Verification items for the finished model (mm, model axes). A direction names the side the tool comes from. Coordinates: 2 decimals unless noted, no trailing zeros. Order: outer loops, then holes, each group sorted by start corner. A loop starts at its lowest first (then second) coordinate and runs counter-clockwise, first axis right, second up. Notation, with made-up numbers: (-27.5, -12.75) -> (24.5, -12.75) arc R16 cw to (24.5, 13.25) -> close; hole circle Ø10 at (56, 72.25). An arc over 180 degrees is marked (long way). Use CSV: the item, a comma, the result in double quotes. Start each with the question number.
1) Tool access check on faces 1 (the flat face through (6, 19.25, 0)), 2 (the flat face through (1, 22, 9)), 3 (the flat face through (0, 10, -3)). Record the directions out of +Z, -Z, +X, -X, +Y, -Y that give a thin tool (end or side, any length) a straight path to the whole face; none if there is none.
2) Sectioned sample at A-A on y = 22.75. Record the boundary of the cut face in (x, z), then the cut area to 3 significant figures.
3) Release check for a two-part mould opening along Y. For faces 4 (the flat face through (4, 1, 0)), 5 (the flat face through (4, 26.25, 0)), 6 (the cylindrical face through (0.986, -9.366, -6.077)) record: released by +Y, released by -Y, zero draft, split by the parting line, or undercut.
4) Sectioned sample at B-B on x = 6. Record the boundary of the cut face in (y, z), then the cut area to 3 significant figures.
5) Sectioned sample at C-C on z = -0.5. Record the boundary of the cut face in (x, y), then the cut area to 3 significant figures.
6) Go/stop test with flat-tipped pins: pin 1 (1.6 mm diameter, centred on y = 23.5, z = -6, fed in from -X); pin 2 (8 mm diameter, centred on y = -9.5, z = 0, fed in from +X) (1 decimal); pin 3 (10 mm diameter, centred on y = 0.5, z = 4, fed in from +X); pin 4 (2 mm diameter, centred on x = 6.5, z = -3.5, fed in from -Y). Record where each tip stops, or that it passes through.
7) Scan lines: line 1 along Y through (x, z) = (5, -7.5); line 2 along Y through (x, z) = (6, 0.5); line 3 along Z through (x, y) = (1.75, 6). Record each from-to range of solid material in increasing order.
8) Sectioned sample at D-D on x = 2.5. Record the boundary of the cut face in (y, z).
from build123d import *

# Parameters (mm, degrees)
SKETCH_1_W                    = 26
SKETCH_1_H                    = 43.75
EXTRUDE_1_DEPTH               = 8
CUT_EXTRUDE_1_DEPTH           = 2
SKETCH_3_W                    = 4
SKETCH_3_H                    = 36.75
CUT_EXTRUDE_2_DEPTH           = 38.802943007
HOLE_WIZARD_M2_51_D           = 3
HOLE_WIZARD_M2_51_CBORE_D     = 5.5
HOLE_WIZARD_M2_51_CBORE_DEPTH = 1
HOLE_WIZARD_9_0_9_1_D         = 9
HOLE_WIZARD_9_0_9_1_DEPTH     = 4
FILLET_1_R                    = 7


with BuildPart() as part:
    # Эскиз1 → Бобышка-Вытянуть1 (new body)
    with BuildSketch(Plane(origin=(8, 0, 0), x_dir=(0, 0, -1), z_dir=(1, 0, 0))):
        with Locations((0, 4.375)):
            Rectangle(SKETCH_1_W, SKETCH_1_H)
    extrude(amount=-EXTRUDE_1_DEPTH)

    # Эскиз2 → Вырез-Вытянуть1 (cut)
    with BuildSketch(Plane.ZY):
        with BuildLine():
            Line((3.901238196, -17.5), (4.545454545, -13.652408939))
            ThreePointArc((4.545454545, -13.652408939), (6.222727273, -9.431365141), (4.545454545, -5.210321344))
            Line((4.545454545, -5.210321344), (2.795454545, 8.289678656))
            ThreePointArc((2.795454545, 8.289678656), (0.072727273, 11.012405929), (-2.65, 8.289678656))
            Line((-2.65, 8.289678656), (-4.4, -5.210321344))
            ThreePointArc((-4.4, -5.210321344), (-6.077272727, -9.431365141), (-4.4, -13.652408939))
            Line((-4.4, -13.652408939), (-3.901238196, -17.5))
            Line((-3.901238196, -17.5), (3.901238196, -17.5))
        make_face()
    extrude(amount=-CUT_EXTRUDE_1_DEPTH, mode=Mode.SUBTRACT)

    # Эскиз3 → Вырез-Вытянуть2 (cut, through all)
    with BuildSketch(Plane.XY.offset(13)):
        with Locations((6, 0.875)):
            Rectangle(SKETCH_3_W, SKETCH_3_H)
    extrude(amount=-CUT_EXTRUDE_2_DEPTH, mode=Mode.SUBTRACT)

    # Цековка для винта с заклепочной головкой M2.51 (through all)
    with Locations(Plane.ZY):
        with Locations((-7.5, 22.75), (7.5, 22.75)):
            CounterBoreHole(HOLE_WIZARD_M2_51_D / 2, HOLE_WIZARD_M2_51_CBORE_D / 2, HOLE_WIZARD_M2_51_CBORE_DEPTH)

    # Диаметр отверстия Ø9.0 (9)1
    with Locations(Plane(origin=(4, 0, 0), x_dir=(0, 0, -1), z_dir=(1, 0, 0))):
        with Locations((0, -9.5)):
            Hole(HOLE_WIZARD_9_0_9_1_D / 2, depth=HOLE_WIZARD_9_0_9_1_DEPTH)

    # Скругление1
    fillet_1_edges = [part.edges().sort_by_distance(p)[0] for p in [
        (2, -17.5, -13),
        (2, -17.5, 13),
    ]]
    fillet(fillet_1_edges, radius=FILLET_1_R)


solid = part.part
Answers follow:
1,face 1,"+Z, -Z, +X, -Y"
1,face 2,"-X"
1,face 3,"+Z, -Z, -X, +Y, -Y"
2,outline,"(0, -13) -> (8, -13) -> (8, -9) -> (1, -9) -> (1, -10.25) -> (0, -10.25) -> close; (0, -4.75) -> (1, -4.75) -> (1, -6) -> (8, -6) -> (8, 6) -> (1, 6) -> (1, 4.75) -> (0, 4.75) -> close; (0, 10.25) -> (1, 10.25) -> (1, 9) -> (8, 9) -> (8, 13) -> (0, 13) -> close"
2,area,"155 mm²"
3,face 4,"zero draft"
3,face 5,"released by +Y"
3,face 6,"undercut"
4,outline,"(19.25, -13) -> (26.25, -13) -> (26.25, 13) -> (19.25, 13) -> close; hole circle Ø3 at (22.75, -7.5); hole circle Ø3 at (22.75, 7.5)"
4,area,"168 mm²"
5,outline,"(0, 10.95) -> (2, 10.95) -> (2, -5.03) -> (4, -5.03) -> (4, 19.25) -> (8, 19.25) -> (8, 26.25) -> (0, 26.25) -> close; (2, -17.5) -> (4, -17.5) -> (4, -13.97) -> (2, -13.97) -> close"
5,area,"128 mm²"
6,pin 1,"stops at x = 1"
6,pin 2,"passes through"
6,pin 3,"stops at x = 4"
6,pin 4,"stops at y = 19.25"
7,line 1,"y = 19.25 to 21.25, 24.25 to 26.25"
7,line 2,"y = 19.25 to 26.25"
7,line 3,"z = -13 to -2.95, 3.09 to 13"
8,outline,"(-17.5, -6) arc R7 ccw to (-10.5, -13) -> (26.25, -13) -> (26.25, 13) -> (-10.5, 13) arc R7 ccw to (-17.5, 6) -> close; hole circle Ø9 at (-9.5, 0); hole circle Ø3 at (22.75, -7.5); hole circle Ø3 at (22.75, 7.5)"
